Part model, mm, in its own coordinate system. Face numbers are marked on the shaded views. A direction names the side the tool comes from. Give positions to 0.01 mm unless a question says otherwise; leave off trailing zeros. Order: outer loops, then holes, each group sorted by start corner. A loop starts at its lowest first (then second) coordinate and runs counter-clockwise, first axis right, second up. Notation, with made-up numbers: (18, -3.5) - (67, -3.5) arc R19 cw to (67, 16.5) - close; hole circle Ø10 at (-27.5, 31.25). An arc over 180 degrees is marked (long way). Use a Markdown table: item, result. Add a question column.
from build123d import *

# Parameters (mm, degrees)
SKETCH2_R   = 4.7625
SKETCH2_R_2 = 3.175


with BuildPart() as part:
    # Sweep2: sweep along a path in Sketch4
    with BuildLine(Plane(origin=(0, 0, 0), x_dir=(0, 0, -1), z_dir=(1, 0, 0))) as sweep2_path:
        Line((8, 0), (8, 10))
        Line((8, 10), (58, 10))
        Line((58, 10), (208, 269.807621135))
        Line((208, 269.807621135), (258, 269.807621135))
    # Sketch2 → Sweep2 (sweep)
    with BuildSketch(Plane(origin=(0, 0, 0), x_dir=(1, 0, 0), z_dir=(0, 1, 0))):
        with Locations((0, 8)):
            Circle(SKETCH2_R)
        with Locations((0, 8)):
            Circle(SKETCH2_R_2, mode=Mode.SUBTRACT)
    sweep(path=sweep2_path.line, transition=Transition.RIGHT)


solid = part.part
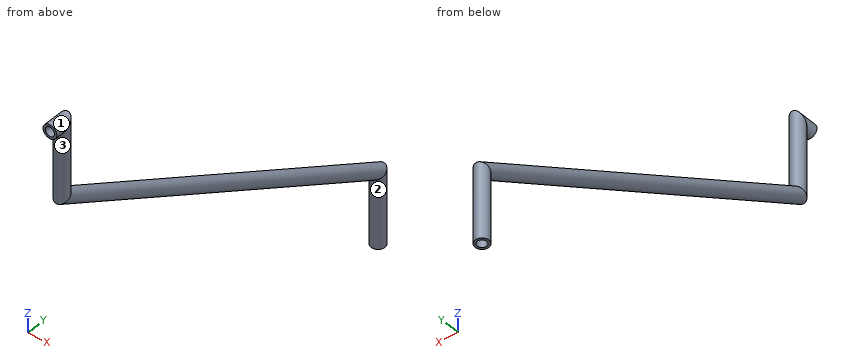
1. Drill centre lines: probe 1 along X at (y, z) = (7.75, -8) (1 decimal); probe 2 along Y at (x, z) = (0, -217.5); probe 3 along Z at (x, y) = (0, 4.5) (1 decimal). Where is each one in solid material? Low to high. Write a range as [from, to].
2. Pin check, flat tips, straight feed: P1, Ø5, axis at x = -1, y = 232.5, coming from the +Z side; P2, Ø5, axis at x = 0, z = -8, coming from the -Y side; P3, Ø1, axis at x = -2, y = 31.5, coming from the +Z side. Stop position of each tip, or through.
3. Cut at A-A (x = 0). Write the cut outline in (y, z) (1 decimal), plus the area to 3 significant figures.
4. Tool access for the marked faces 1, 2 and 3: list every direction of +Z, -Z, +X, -X, +Y, -Y with a clear straight run to the whole face (end or side of a thin tool).
Responses:
| question | item | result |
|---|---|---|
| 1 | probe 1 | x = [-4.8, -3.2], [3.2, 4.8] |
| 1 | probe 2 | y = [265.05, 266.63], [272.98, 274.57] |
| 1 | probe 3 | z = [-12.8, -11.2], [-4.8, -3.2] |
| 2 | P1 | stops at z = -179.58 |
| 2 | P2 | stops at y = 11.96 |
| 2 | P3 | stops at z = -65.05 |
| 3 | outline | (0, -12.8) - (5.2, -12.8) - (5.2, -60.7) - (265, -210.7) - (265, -258) - (266.6, -258) - (266.6, -209.8) - (6.8, -59.8) - (6.8, -11.2) - (0, -11.2) - close; (0, -4.8) - (13.2, -4.8) - (13.2, -56.2) - (273, -206.2) - (273, -258) - (274.6, -258) - (274.6, -205.3) - (14.8, -55.3) - (14.8, -3.2) - (0, -3.2) - close |
| 3 | area | 1,300 mm² |
| 4 | face 1 | -Y |
| 4 | face 2 | -Z |
| 4 | face 3 | none |
